Here's how the part is built. I have some questions about the finished solid (model axes, mm). Face numbers are marked on the shaded views. A direction names the side the tool comes from. Round coordinates to 2 decimals unless told otherwise and drop trailing zeros. Use one line per item in the form item = value. Start each with the question number.
Q1. We'd pull the mould along Z, two halves only. Please class the marked faces 3, 4, 5 and 6: +Z half, -Z half, draft (parallel to the pull), parting line (faces both ways), or undercut.
Q2. I want a section at A-A on z = -39.5. State how many separate pieces and enclosed holes the cut face has, and give its area (3 significant figures).
Q3. I'm going to push flat-ended pins straight in: pin 1 Ø4 at (x, y) = (-61.5, 9.5) entering from -Z; pin 2 Ø6 at (x, z) = (61.16, -25.33) entering from -Y; pin 3 Ø4 at (x, y) = (14, 6) entering from -Z; pin 4 Ø1 at (x, y) = (45.5, 8) entering from +Z. Where does each tip first touch, or does it pass through?
Q4. For the marked faces 1 and 2, which set-ups out of +Z, -Z, +X, -X, +Y, -Y let a thin tool reach every point of the face, with its end or its side?
Q5. I need wall thicknesses on line 1 along Z through (x, y) = (0, 3.5); line 2 along X through (y, z) = (0.5, -52.5); line 3 along Z through (x, y) = (-51, 6.5). Which ranges of each line are inside material? Lowest first, please. Write a range as from..to.
```python
from build123d import *

# Parameters (mm, degrees)
SKETCH2_W                   = 77.55
SKETCH2_H                   = 12.7
F_12_0_189_DIAMETER_HOLE1_D = 4.8006
CIRPATTERN3_COUNT           = 4
CUT_EXTRUDE1_DEPTH          = 13.7
FILLET1_R                   = 4
CIRPATTERN4_COUNT           = 8
FILLET1_OF_CIRPATTERN4_R    = 4
CHAMFER1_SIZE               = 1
SKETCH15_W                  = 2.0447
SKETCH15_H                  = 101.323957926
SKETCH19_R                  = 6.25
CUT_EXTRUDE3_DEPTH          = 5
CIRPATTERN5_COUNT           = 2
CIRPATTERN6_COUNT           = 2
SKETCH22_R                  = 3.96875
CUT_EXTRUDE4_DEPTH          = 12.8


with BuildPart() as part:
    # Sketch2 → Revolve1 (revolve)
    with BuildSketch(Plane(origin=(0, 0, 0), x_dir=(0, 0, -1), z_dir=(1, 0, 0))):
        with Locations((-38.775, 6.35)):
            Rectangle(SKETCH2_W, SKETCH2_H)
    revolve(axis=Axis((0, -0.888756804, 0), (0, 1, 0)))

    # #12 (0.189) Diameter Hole1 (through all)
    with Locations(Plane(origin=(0, 12.7, 0), x_dir=(1, 0, 0), z_dir=(0, 1, 0))):
        with Locations((-25.333643223, 61.160825052)):
            f_12_0_189_diameter_hole1 = Hole(F_12_0_189_DIAMETER_HOLE1_D / 2)

    # CirPattern3: #12 (0.189) Diameter Hole1 ×4 about axis
    cirpattern3_axis = Axis((0, 0, 0), (0, 1, 0))
    for i in range(1, CIRPATTERN3_COUNT):
        add(f_12_0_189_diameter_hole1.rotate(cirpattern3_axis, i * 360 / CIRPATTERN3_COUNT), mode=Mode.SUBTRACT)

    # Sketch8 → Cut-Extrude1 (cut, through all)
    with BuildSketch(Plane(origin=(0, 12.7, 0), x_dir=(1, 0, 0), z_dir=(0, 1, 0))):
        with BuildLine():
            Line((-17.167098173, 54.510670885), (-21.735525784, 65.539830782))
            ThreePointArc((-21.735525784, 65.539830782), (0, 69.05), (21.735525784, 65.539830782))
            Line((21.735525784, 65.539830782), (17.167098173, 54.510670885))
            ThreePointArc((17.167098173, 54.510670885), (0, 57.15), (-17.167098173, 54.510670885))
        make_face()
    cut_extrude1 = extrude(amount=-CUT_EXTRUDE1_DEPTH, mode=Mode.SUBTRACT)

    # Fillet1
    fillet1_edges = [part.edges().sort_by_distance(p)[0] for p in [
        (17.167098173, 6.35, -54.510670885),
        (-17.167098173, 6.35, -54.510670885),
        (-21.735525784, 6.35, -65.539830782),
        (21.735525784, 6.35, -65.539830782),
    ]]
    fillet(fillet1_edges, radius=FILLET1_R)

    # CirPattern4: Cut-Extrude1 ×8 about axis
    cirpattern4_axis = Axis((0, 0, 0), (0, 1, 0))
    for i in range(1, CIRPATTERN4_COUNT):
        add(cut_extrude1.rotate(cirpattern4_axis, i * 360 / CIRPATTERN4_COUNT), mode=Mode.SUBTRACT)

    # Fillet1 of CirPattern4
    fillet1_of_cirpattern4_edges = [part.edges().sort_by_distance(p)[0] for p in [
        (-26.405893498, 6.35, -50.683836561),
        (-50.683836561, 6.35, -26.405893498),
        (-61.712996458, 6.35, -30.974321109),
        (-30.974321109, 6.35, -61.712996458),
        (-54.510670885, 6.35, -17.167098173),
        (-54.510670885, 6.35, 17.167098173),
        (-65.539830782, 6.35, 21.735525784),
        (-65.539830782, 6.35, -21.735525784),
        (-50.683836561, 6.35, 26.405893498),
        (-26.405893498, 6.35, 50.683836561),
        (-30.974321109, 6.35, 61.712996458),
        (-61.712996458, 6.35, 30.974321109),
        (-17.167098173, 6.35, 54.510670885),
        (17.167098173, 6.35, 54.510670885),
        (21.735525784, 6.35, 65.539830782),
        (-21.735525784, 6.35, 65.539830782),
        (26.405893498, 6.35, 50.683836561),
        (50.683836561, 6.35, 26.405893498),
        (61.712996458, 6.35, 30.974321109),
        (30.974321109, 6.35, 61.712996458),
        (54.510670885, 6.35, 17.167098173),
        (54.510670885, 6.35, -17.167098173),
        (65.539830782, 6.35, -21.735525784),
        (65.539830782, 6.35, 21.735525784),
        (50.683836561, 6.35, -26.405893498),
        (26.405893498, 6.35, -50.683836561),
        (30.974321109, 6.35, -61.712996458),
        (61.712996458, 6.35, -30.974321109),
    ]]
    fillet(fillet1_of_cirpattern4_edges, radius=FILLET1_OF_CIRPATTERN4_R)

    # Chamfer1
    chamfer1_edges = [part.edges().sort_by_distance(p)[0] for p in [
        (0, 12.7, -77.55),
        (0, 0, -77.55),
    ]]
    chamfer(chamfer1_edges, length=CHAMFER1_SIZE)

    # Sketch15 → #20 (0.161) Diameter Hole1 (revolve, cut)
    with BuildSketch(Plane(origin=(0, 6.35, 0), x_dir=(-0.382683432, 0, 0.923879533), z_dir=(0, 1, 0))):
        with Locations((1.02235, 50.661978963)):
            Rectangle(SKETCH15_W, SKETCH15_H)
    revolve(axis=Axis((-5.866635031, 6.35, -2.430039796), (0.923879533, 0, 0.382683432)), mode=Mode.SUBTRACT)

    # Sketch19 → Cut-Extrude3 (cut)
    with BuildSketch(Plane(origin=(29.67710018, 0, -71.646857746), x_dir=(-0.923879533, 0, -0.382683432), z_dir=(0.382683432, 0, -0.923879533))):
        with Locations((0, 6.35)):
            Circle(SKETCH19_R)
    cut_extrude3 = extrude(amount=-CUT_EXTRUDE3_DEPTH, mode=Mode.SUBTRACT)

    # CirPattern5: Cut-Extrude3 ×2 about axis
    cirpattern5_axis = Axis((0, -0.888756804, 0), (0, 1, 0))
    for i in range(1, CIRPATTERN5_COUNT):
        add(cut_extrude3.rotate(cirpattern5_axis, i * 360 / CIRPATTERN5_COUNT), mode=Mode.SUBTRACT)

    # Sketch21 → #10-24 Tapped Hole1 (revolve, cut)
    with BuildSketch(Plane(origin=(-27.763683018, 6.35, 67.027460084), x_dir=(0.923879533, 0, 0.382683432), z_dir=(0, 1, 0))):
        Polygon((0, 0), (0, 51.940824014), (1.89865, 50.8), (1.89865, 0), align=None)
    f_10_24_tapped_hole1 = revolve(axis=Axis((-30.193722814, 6.35, 72.894095115), (0.382683432, 0, -0.923879533)), mode=Mode.SUBTRACT)

    # CirPattern6: #10-24 Tapped Hole1 ×2 about axis
    cirpattern6_axis = Axis((0, -0.888756804, 0), (0, 1, 0))
    for i in range(1, CIRPATTERN6_COUNT):
        add(f_10_24_tapped_hole1.rotate(cirpattern6_axis, i * 360 / CIRPATTERN6_COUNT), mode=Mode.SUBTRACT)

    # Sketch22 → Cut-Extrude4 (cut)
    with BuildSketch(Plane(origin=(0, 12.7, 0), x_dir=(1, 0, 0), z_dir=(0, 1, 0))):
        Circle(SKETCH22_R)
    extrude(amount=-CUT_EXTRUDE4_DEPTH, mode=Mode.SUBTRACT)


solid = part.part
```
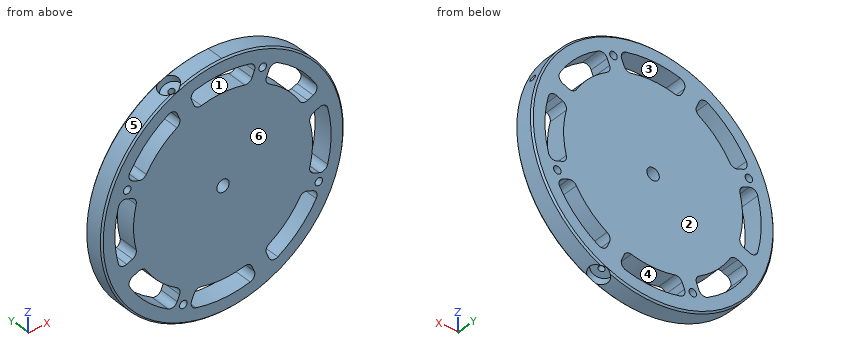
Reported:
q1.face_3 = undercut
q1.face_4 = undercut
q1.face_5 = parting line
q1.face_6 = draft
q2.separate_pieces = 3
q2.enclosed_holes = 1
q2.area = 1,290 mm^2
q3.pin_1 = -49.74
q3.pin_2 = 0
q3.pin_3 = -76.62
q3.pin_4 = 63.16
q4.face_1 = +Y, -Y
q4.face_2 = +Z, -Z, +X, -X, +Y
q5.line_1 = -77.55..-69.05, -57.15..-3.97, 3.97..57.15, 69.05..77.55
q5.line_2 = -56.4..-44.85, -27.46..27.46, 44.85..56.4
q5.line_3 = -58.42..-46.55, -27.73..27.73, 46.55..58.42
